```python
from build123d import *

# Parameters (mm, degrees)
SKETCH1_R           = 25
SKETCH1_R_2         = 1.75
BOSS_EXTRUDE1_DEPTH = 4
SKETCH2_W           = 27.5
SKETCH2_H           = 30
BOSS_EXTRUDE2_DEPTH = 50
CUT_EXTRUDE1_DEPTH  = 41
SKETCH4_W           = 17
SKETCH4_H           = 46
CUT_EXTRUDE2_DEPTH  = 24.5
CUT_EXTRUDE3_REACH  = 16.25
SKETCH5_R           = 1.75
SKETCH5_W           = 14.1
SKETCH5_H           = 34.1


with BuildPart() as part:
    # Sketch1 → Boss-Extrude1 (new body)
    with BuildSketch(Plane(origin=(0, 0, 0), x_dir=(1, 0, 0), z_dir=(0, 1, 0))):
        Circle(SKETCH1_R)
        with Locations((-17.320508076, 10)):
            Circle(SKETCH1_R_2, mode=Mode.SUBTRACT)
        with Locations((17.320508076, 10)):
            Circle(SKETCH1_R_2, mode=Mode.SUBTRACT)
        with Locations((17.320508076, -10)):
            Circle(SKETCH1_R_2, mode=Mode.SUBTRACT)
        with Locations((-17.320508076, -10)):
            Circle(SKETCH1_R_2, mode=Mode.SUBTRACT)
    extrude(amount=BOSS_EXTRUDE1_DEPTH)

    # Sketch2 → Boss-Extrude2 (add)
    with BuildSketch(Plane(origin=(0, 4, 0), x_dir=(1, 0, 0), z_dir=(0, 1, 0))):
        Rectangle(SKETCH2_W, SKETCH2_H)
    extrude(amount=BOSS_EXTRUDE2_DEPTH)

    # Sketch3 → Cut-Extrude1 (cut, through all)
    with BuildSketch(Plane.XY.offset(15)):
        with BuildLine():
            ThreePointArc((2.439273587, 50.792164924), (4.647822502, 53.135805173), (7.75, 54))
            Line((7.75, 54), (-13.75, 54))
            Line((-13.75, 54), (-13.75, 20))
            Line((-13.75, 20), (2.439273587, 50.792164924))
        make_face()
        with BuildLine():
            Line((13.75, 48), (13.75, 54))
            Line((13.75, 54), (7.75, 54))
            ThreePointArc((7.75, 54), (11.992640687, 52.242640687), (13.75, 48))
        make_face()
    extrude(amount=-CUT_EXTRUDE1_DEPTH, mode=Mode.SUBTRACT)

    # Sketch4 → Cut-Extrude2 (cut)
    with BuildSketch(Plane.ZY.offset(13.75)):
        with Locations((0, 27.792164924)):
            Rectangle(SKETCH4_W, SKETCH4_H)
    extrude(amount=-CUT_EXTRUDE2_DEPTH, mode=Mode.SUBTRACT)

    # Sketch5 → Cut-Extrude3 (cut, up to next)
    with BuildSketch(Plane.ZY.offset(-10.75), mode=Mode.PRIVATE) as cut_extrude3_sk1:
        with Locations((-4.55, 47.802164924)):
            Circle(SKETCH5_R)
    cut_extrude3_tool1 = extrude(cut_extrude3_sk1.sketch, amount=-CUT_EXTRUDE3_REACH, mode=Mode.PRIVATE) & part.part
    add(cut_extrude3_tool1.solids().sort_by_distance((10.75, 47.802165, -4.55))[0], mode=Mode.SUBTRACT)
    # Sketch5 → Cut-Extrude3 (cut, up to next)
    with BuildSketch(Plane.ZY.offset(-10.75), mode=Mode.PRIVATE) as cut_extrude3_sk2:
        with Locations((-4.55, 7.782164924)):
            Circle(SKETCH5_R)
    cut_extrude3_tool2 = extrude(cut_extrude3_sk2.sketch, amount=-CUT_EXTRUDE3_REACH, mode=Mode.PRIVATE) & part.part
    add(cut_extrude3_tool2.solids().sort_by_distance((10.75, 7.782165, -4.55))[0], mode=Mode.SUBTRACT)
    # Sketch5 → Cut-Extrude3 (cut, up to next)
    with BuildSketch(Plane.ZY.offset(-10.75), mode=Mode.PRIVATE) as cut_extrude3_sk3:
        with Locations((4.55, 7.782164924)):
            Circle(SKETCH5_R)
    cut_extrude3_tool3 = extrude(cut_extrude3_sk3.sketch, amount=-CUT_EXTRUDE3_REACH, mode=Mode.PRIVATE) & part.part
    add(cut_extrude3_tool3.solids().sort_by_distance((10.75, 7.782165, 4.55))[0], mode=Mode.SUBTRACT)
    # Sketch5 → Cut-Extrude3 (cut, up to next)
    with BuildSketch(Plane.ZY.offset(-10.75), mode=Mode.PRIVATE) as cut_extrude3_sk4:
        with Locations((4.55, 47.802164924)):
            Circle(SKETCH5_R)
    cut_extrude3_tool4 = extrude(cut_extrude3_sk4.sketch, amount=-CUT_EXTRUDE3_REACH, mode=Mode.PRIVATE) & part.part
    add(cut_extrude3_tool4.solids().sort_by_distance((10.75, 47.802165, 4.55))[0], mode=Mode.SUBTRACT)
    # Sketch5 → Cut-Extrude3 (cut, up to next)
    with BuildSketch(Plane.ZY.offset(-10.75), mode=Mode.PRIVATE) as cut_extrude3_sk5:
        with Locations((0, 27.792164924)):
            Rectangle(SKETCH5_W, SKETCH5_H)
    cut_extrude3_tool5 = extrude(cut_extrude3_sk5.sketch, amount=-CUT_EXTRUDE3_REACH, mode=Mode.PRIVATE) & part.part
    add(cut_extrude3_tool5.solids().sort_by_distance((10.75, 27.792165, 0))[0], mode=Mode.SUBTRACT)


solid = part.part
```
Read the model definition and answer for the solid it produces. Units are mm, in the model's axes. A direction names the side the tool comes from. Round coordinates to 2 decimals unless told otherwise and drop trailing zeros. Write each loop counter-clockwise with the first axis right and the second up, starting at its lowest first coordinate (ties: lowest second). Pieces come first, ordered by that corner, then holes. Notation, with made-up numbers: (80, -13) -> (132, -13) arc R31 cw to (132, 23) -> close; hole circle Ø10 at (-19.75, 58). An arc over 180 degrees is marked (long way). Answer in a Markdown table with one row per item. Add a question column.
1) Given P1, Ø5.5, axis at y = 7.78, z = 4.55, coming from the +X side; P2, Ø3, axis at x = 18, z = 7.5, coming from the +Y side; P3, Ø12, axis at x = -5, y = 14.5, coming from the +Z side; P4, Ø3, axis at x = -17.32, z = 10, coming from the +Y side, each flat-ended and moving along its own axis, determine where each tip first touches the part or whether it passes through.
2) Find section B-B, the plane y = 39. Determine the outline of the cut face in (x, z), and give its area (3 significant figures).
3) Consider line 1 (Z direction, x = -3.5, y = 5); line 2 (Y direction, x = 12, z = 4); line 3 (X direction, y = 1, z = 10). Determine where each line is inside the solid, lowest interval first.
4) Find section D-D, the plane x = 12. Determine the outline of the cut face in (y, z).
5) Find section A-A, the plane z = 1. Determine the outline of the cut face in (x, y).
6) Find section C-C, the plane y = 8.5. Determine the outline of the cut face in (x, z).
7) Which of the six approach directions +Z, -Z, +X, -X, +Y, -Y give full straight-line access (tool end or side, diameter ignored) to faces 4 (the face through (12, 28, 7.05)), 5 (the face through (10.75, 30, -8)), 6 (the face through (-13.75, 12, 10)), 7 (the face through (13.75, 26, 10))?
8) Determine the mould class of faces 1 (the face through (12.229, 46.094, -4.929)), 2 (the face through (3, 23, -15)), 3 (the face through (16, 4, 0)) for opening direction Z: pulls with the +Z half, pulls with the -Z half, needs draft (parallel to the pull), parting line crosses it, or undercut.
Findings below:
| question | item | result |
|---|---|---|
| 1 | P1 | x = 13.75 |
| 1 | P2 | y = 4 |
| 1 | P3 | z = 15 |
| 1 | P4 | through |
| 2 | outline | (-3.76, -15) -> (13.75, -15) -> (13.75, -7.05) -> (10.75, -7.05) -> (10.75, -8.5) -> (-3.76, -8.5) -> close; (-3.76, 8.5) -> (10.75, 8.5) -> (10.75, 7.05) -> (13.75, 7.05) -> (13.75, 15) -> (-3.76, 15) -> close |
| 2 | area | 236 mm² |
| 3 | line 1 | -15 to -8.5, 8.5 to 15 |
| 3 | line 2 | 0 to 6.12, 9.44 to 10.74, 44.84 to 46.14, 49.46 to 52.24 |
| 3 | line 3 | -22.91 to -19.07, -15.57 to 15.57, 19.07 to 22.91 |
| 4 | outline | (0, -21.93) -> (4, -21.93) -> (4, -15) -> (52.24, -15) -> (52.24, 15) -> (4, 15) -> (4, 21.93) -> (0, 21.93) -> close; hole circle Ø3.5 at (7.78, -4.55); hole circle Ø3.5 at (7.78, 4.55); hole (10.74, -7.05) -> (44.84, -7.05) -> (44.84, 7.05) -> (10.74, 7.05) -> close; hole circle Ø3.5 at (47.8, -4.55); hole circle Ø3.5 at (47.8, 4.55) |
| 5 | outline | (-24.98, 0) -> (24.98, 0) -> (24.98, 4) -> (13.75, 4) -> (13.75, 10.74) -> (10.75, 10.74) -> (10.75, 4.79) -> (-13.75, 4.79) -> (-13.75, 4) -> (-24.98, 4) -> close; (2.44, 50.79) -> (10.75, 50.79) -> (10.75, 44.84) -> (13.75, 44.84) -> (13.75, 48) arc R6 ccw to start |
| 6 | outline | (-13.75, -15) -> (13.75, -15) -> (13.75, -6.15) -> (10.75, -6.15) -> (10.75, -8.5) -> (-13.75, -8.5) -> close; (-13.75, 8.5) -> (10.75, 8.5) -> (10.75, 6.15) -> (13.75, 6.15) -> (13.75, 15) -> (-13.75, 15) -> close; (10.75, -2.95) -> (13.75, -2.95) -> (13.75, 2.95) -> (10.75, 2.95) -> close |
| 7 | face 4 | +X, -X |
| 7 | face 5 | -X |
| 7 | face 6 | +Z, -Z, -X, +Y |
| 7 | face 7 | +Z, -Z, +X, +Y |
| 8 | face 1 | undercut |
| 8 | face 2 | pulls with the -Z half |
| 8 | face 3 | needs draft |
